from build123d import *

# Parameters (mm, degrees)
SKETCH1_R            = 3
SKETCH1_R_2          = 1.5
BOSS_EXTRUDE1_DEPTH  = 1.7
SKETCH4_W            = 49.75
SKETCH4_H            = 5.233449475
BOSS_EXTRUDE4_DEPTH  = 3
SKETCH7_W            = 6.5
SKETCH7_H            = 5.5
SKETCH7_W_2          = 7
SKETCH7_H_2          = 0.5
BOSS_EXTRUDE7_DEPTH  = 3
SKETCH8_W            = 13
SKETCH8_H            = 12
BOSS_EXTRUDE8_DEPTH  = 6.5
SKETCH9_W            = 5
SKETCH9_H            = 12
BOSS_EXTRUDE9_DEPTH  = 6
SKETCH10_W           = 20
SKETCH10_H           = 14
BOSS_EXTRUDE10_DEPTH = 13.5
SKETCH11_W           = 17
SKETCH11_H           = 12
BOSS_EXTRUDE11_DEPTH = 16
SKETCH12_W           = 10.053569384
SKETCH12_H           = 13.342225903
SKETCH12_W_2         = 14.279787724
SKETCH12_H_2         = 14.279787724
SKETCH12_W_3         = 9
SKETCH12_H_3         = 9
BOSS_EXTRUDE12_DEPTH = 2
SKETCH13_R           = 2.25
SKETCH13_R_2         = 1.5
BOSS_EXTRUDE13_DEPTH = 2
CUT_EXTRUDE1_DEPTH   = 9
CUT_EXTRUDE2_DEPTH   = 5
SKETCH16_W           = 11
SKETCH16_H           = 4
CUT_EXTRUDE3_DEPTH   = 10
SKETCH17_W           = 11
SKETCH17_H           = 4
CUT_EXTRUDE4_DEPTH   = 10
CUT_EXTRUDE5_DEPTH   = 12


with BuildPart() as part:
    # Sketch1 → Boss-Extrude1 (new body)
    with BuildSketch(Plane(origin=(0, 0, 0), x_dir=(1, 0, 0), z_dir=(0, 1, 0))):
        with BuildLine():
            ThreePointArc((39.5, 24.5), (41.621320344, 23.621320344), (42.5, 21.5))
            Line((42.5, 21.5), (42.5, -28.5))
            ThreePointArc((42.5, -28.5), (41.621320344, -30.621320344), (39.5, -31.5))
            Line((39.5, -31.5), (-39.5, -31.5))
            ThreePointArc((-39.5, -31.5), (-41.621320344, -30.621320344), (-42.5, -28.5))
            Line((-42.5, -28.5), (-42.5, 21.5))
            ThreePointArc((-42.5, 21.5), (-41.621320344, 23.621320344), (-39.5, 24.5))
            Line((-39.5, 24.5), (39.5, 24.5))
        make_face()
        with Locations((19, -28)):
            Circle(SKETCH1_R, mode=Mode.SUBTRACT)
        with Locations((19, 21)):
            Circle(SKETCH1_R, mode=Mode.SUBTRACT)
        with Locations((-39, -28)):
            Circle(SKETCH1_R, mode=Mode.SUBTRACT)
        with Locations((-39, 21)):
            Circle(SKETCH1_R, mode=Mode.SUBTRACT)
        with Locations((19, 21)):
            Circle(SKETCH1_R)
        with Locations((19, 21)):
            Circle(SKETCH1_R_2, mode=Mode.SUBTRACT)
        with Locations((-39, 21)):
            Circle(SKETCH1_R)
        with Locations((-39, 21)):
            Circle(SKETCH1_R_2, mode=Mode.SUBTRACT)
        with Locations((-39, -28)):
            Circle(SKETCH1_R)
        with Locations((-39, -28)):
            Circle(SKETCH1_R_2, mode=Mode.SUBTRACT)
        with Locations((19, -28)):
            Circle(SKETCH1_R)
        with Locations((19, -28)):
            Circle(SKETCH1_R_2, mode=Mode.SUBTRACT)
    extrude(amount=BOSS_EXTRUDE1_DEPTH)

    # Sketch4 → Boss-Extrude4 (add)
    with BuildSketch(Plane(origin=(0, 1.7, 0), x_dir=(1, 0, 0), z_dir=(0, 1, 0))):
        with Locations((-10, 21.068102783)):
            Rectangle(SKETCH4_W, SKETCH4_H)
    extrude(amount=BOSS_EXTRUDE4_DEPTH)

    # Sketch7 → Boss-Extrude7 (add)
    with BuildSketch(Plane(origin=(0, 1.7, 0), x_dir=(1, 0, 0), z_dir=(0, 1, 0))):
        with Locations((-31.9, -29.194183223)):
            Rectangle(SKETCH7_W, SKETCH7_H)
        with Locations((-31.9, -32.194183223)):
            Rectangle(SKETCH7_W_2, SKETCH7_H_2)
    extrude(amount=BOSS_EXTRUDE7_DEPTH)

    # Sketch8 → Boss-Extrude8 (add)
    with BuildSketch(Plane(origin=(0, 1.7, 0), x_dir=(1, 0, 0), z_dir=(0, 1, 0))):
        with Locations((-10.5, -26.626453528)):
            Rectangle(SKETCH8_W, SKETCH8_H)
    extrude(amount=BOSS_EXTRUDE8_DEPTH)

    # Sketch9 → Boss-Extrude9 (add)
    with BuildSketch(Plane(origin=(0, 1.7, 0), x_dir=(1, 0, 0), z_dir=(0, 1, 0))):
        with Locations((11, -25.5)):
            Rectangle(SKETCH9_W, SKETCH9_H)
    extrude(amount=BOSS_EXTRUDE9_DEPTH)

    # Sketch10 → Boss-Extrude10 (add)
    with BuildSketch(Plane(origin=(0, 1.7, 0), x_dir=(1, 0, 0), z_dir=(0, 1, 0))):
        with Locations((35, -21.25)):
            Rectangle(SKETCH10_W, SKETCH10_H)
    extrude(amount=BOSS_EXTRUDE10_DEPTH)

    # Sketch11 → Boss-Extrude11 (add)
    with BuildSketch(Plane(origin=(0, 1.7, 0), x_dir=(1, 0, 0), z_dir=(0, 1, 0))):
        with Locations((36.5, -2.5)):
            Rectangle(SKETCH11_W, SKETCH11_H)
        with Locations((36.5, 15.5)):
            Rectangle(SKETCH11_W, SKETCH11_H)
    extrude(amount=BOSS_EXTRUDE11_DEPTH)

    # Sketch12 → Boss-Extrude12 (add)
    with BuildSketch(Plane(origin=(0, 1.7, 0), x_dir=(1, 0, 0), z_dir=(0, 1, 0))):
        with Locations((-29.848215308, 10.97382243)):
            Rectangle(SKETCH12_W, SKETCH12_H)
        with Locations((-15.157331854, -3.918986484)):
            Rectangle(SKETCH12_W_2, SKETCH12_H_2)
        with Locations((19.1, -3.31)):
            Rectangle(SKETCH12_W_3, SKETCH12_H_3)
    extrude(amount=BOSS_EXTRUDE12_DEPTH)

    # Sketch13 → Boss-Extrude13 (add)
    with BuildSketch(Plane.XY.offset(31.5)):
        with Locations((11, 4.7)):
            Circle(SKETCH13_R)
        with Locations((11, 4.7)):
            Circle(SKETCH13_R_2, mode=Mode.SUBTRACT)
    extrude(amount=BOSS_EXTRUDE13_DEPTH)

    # Sketch14 → Cut-Extrude1 (cut)
    with BuildSketch(Plane.XY.offset(32.626453528)):
        with BuildLine():
            Line((-15.750323675, 5.983842352), (-4.86762122, 5.983842352))
            ThreePointArc((-4.86762122, 5.983842352), (-4.705559797, 5.901043441), (-4.677683467, 5.721203306))
            Line((-4.677683467, 5.721203306), (-5.276717124, 3.904778668))
            ThreePointArc((-5.276717124, 3.904778668), (-5.349453787, 3.805356292), (-5.466654877, 3.767417714))
            Line((-5.466654877, 3.767417714), (-15.151290018, 3.767417714))
            ThreePointArc((-15.151290018, 3.767417714), (-15.268491107, 3.805356292), (-15.341227771, 3.904778668))
            Line((-15.341227771, 3.904778668), (-15.940261428, 5.721203306))
            ThreePointArc((-15.940261428, 5.721203306), (-15.912385097, 5.901043441), (-15.750323675, 5.983842352))
        make_face()
    extrude(amount=-CUT_EXTRUDE1_DEPTH, mode=Mode.SUBTRACT)

    # Sketch15 → Cut-Extrude2 (cut)
    with BuildSketch(Plane.XY.offset(32.444183223)):
        with BuildLine():
            Line((-34.475250903, 3.20419671), (-29.43081526, 3.20419671))
            ThreePointArc((-29.43081526, 3.20419671), (-29.27664987, 3.131605628), (-29.234394805, 2.966527034))
            Line((-29.234394805, 2.966527034), (-29.471007813, 1.732759202))
            ThreePointArc((-29.471007813, 1.732759202), (-29.540019351, 1.616263488), (-29.667428269, 1.570428878))
            Line((-29.667428269, 1.570428878), (-34.24114908, 1.570428878))
            ThreePointArc((-34.24114908, 1.570428878), (-34.36870932, 1.616388672), (-34.437643137, 1.733145027))
            Line((-34.437643137, 1.733145027), (-34.67174496, 2.966912859))
            ThreePointArc((-34.67174496, 2.966912859), (-34.62929111, 3.13175695), (-34.475250903, 3.20419671))
        make_face()
    extrude(amount=-CUT_EXTRUDE2_DEPTH, mode=Mode.SUBTRACT)

    # Sketch16 → Cut-Extrude3 (cut)
    with BuildSketch(Plane(origin=(45, 0, 0), x_dir=(0, 0, -1), z_dir=(1, 0, 0))):
        with Locations((-2.5, 4.7)):
            Rectangle(SKETCH16_W, SKETCH16_H)
        with Locations((-2.5, 14.7)):
            Rectangle(SKETCH16_W, SKETCH16_H)
    extrude(amount=-CUT_EXTRUDE3_DEPTH, mode=Mode.SUBTRACT)

    # Sketch17 → Cut-Extrude4 (cut)
    with BuildSketch(Plane(origin=(45, 0, 0), x_dir=(0, 0, -1), z_dir=(1, 0, 0))):
        with Locations((15.5, 14.7)):
            Rectangle(SKETCH17_W, SKETCH17_H)
        with Locations((15.5, 4.7)):
            Rectangle(SKETCH17_W, SKETCH17_H)
    extrude(amount=-CUT_EXTRUDE4_DEPTH, mode=Mode.SUBTRACT)

    # Sketch18 → Cut-Extrude5 (cut)
    with BuildSketch(Plane(origin=(45, 0, 0), x_dir=(0, 0, -1), z_dir=(1, 0, 0))):
        Polygon((-26.75, 14), (-26.75, 3.95), (-23.25, 3.95), (-23.25, 1.95), (-19.25, 1.95), (-19.25, 3.95), (-15.75, 3.95), (-15.75, 14), align=None)
    extrude(amount=-CUT_EXTRUDE5_DEPTH, mode=Mode.SUBTRACT)


solid = part.part
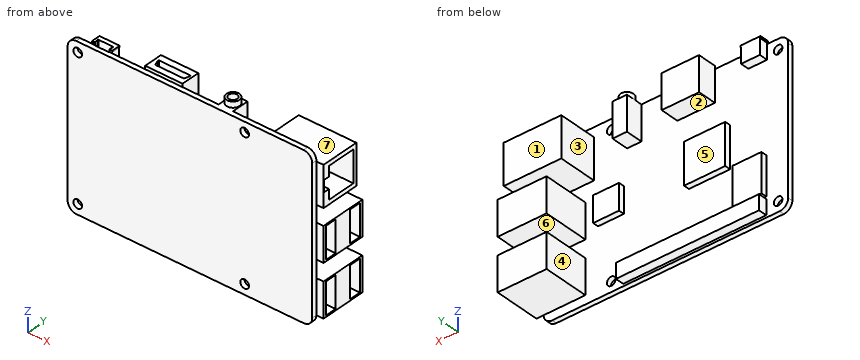
Geometry check sheet. Reference: the model listing, model coordinates, mm. Face numbers are marked on the shaded views. A direction names the side the tool comes from. Give positions to 0.01 mm unless a question says otherwise; leave off trailing zeros. Order: outer loops, then holes, each group sorted by start corner. A loop starts at its lowest first (then second) coordinate and runs counter-clockwise, first axis right, second up. Notation, with made-up numbers: (68, 35.25) - (84, 35.25) arc R16 ccw to (84, 42.25) - close; hole circle Ø3 at (37, 8.5). An arc over 180 degrees is marked (long way). Use one line per item in the form item = value.
1) Sectioned sample at A-A (y = 10.75). Record the boundary of the cut face in (x, z), and give its area (3 significant figures).
Working result:
outline = (25, 14.25) - (45, 14.25) - (45, 15.75) - (33, 15.75) - (33, 26.75) - (45, 26.75) - (45, 28.25) - (25, 28.25) - close; (28, -21.5) - (45, -21.5) - (45, -9.5) - (28, -9.5) - close; (28, -3.5) - (45, -3.5) - (45, 8.5) - (28, 8.5) - close
area = 556 mm^2
2) Sectioned sample at C-C (z = -8.5). Record the boundary of the cut face in (x, y) (3 decimals), and give its area (3 significant figures).
Working result:
outline = (-42.5, 0) - (42.5, 0) - (42.5, 1.7) - (-24.821, 1.7) - (-24.821, 3.7) - (-34.875, 3.7) - (-34.875, 1.7) - (-42.5, 1.7) - close
area = 165 mm^2
3) Depth check by flat-ended pin: pin 1 Ø4.5 at (x, z) = (-13, 2.5) entering from +Y; pin 2 Ø4.5 at (x, y) = (40, 14.5) entering from -Z; pin 3 Ø2 at (y, z) = (5.5, 1) entering from +X. Enter the tip coordinate at first touch or a pass-through.
Working result:
pin_1 = 3.7
pin_2 = -21.5
pin_3 = 35
4) Draft check along Z on the marked faces 4, 5, 6 and 7. Enter one of: released by +Z, released by -Z, zero draft, split by the parting line, or undercut.
Working result:
face_4 = zero draft
face_5 = undercut
face_6 = undercut
face_7 = released by +Z
5) Material ranges on probe 1 along Z at (x, y) = (-39, 0.65); probe 2 along Z at (x, y) = (40, 13); probe 3 along Z at (x, y) = (33, 15), recorded low to high. Write a range as from..to.
Working result:
probe_1 = -24.5..-22.5, -19.5..26.5, 29.5..31.5
probe_2 = -21.5..-21, -10..-9.5, -3.5..-3, 8..8.5, 14.25..15.75, 26.75..28.25
probe_3 = -21.5..-9.5, -3.5..8.5, 14.25..28.25
6) Sectioned sample at B-B (z = 24.5). Record the boundary of the cut face in (x, y).
Working result:
outline = (-42.5, 0) - (42.5, 0) - (42.5, 1.7) - (45, 1.7) - (45, 3.95) - (33, 3.95) - (33, 14) - (45, 14) - (45, 15.2) - (25, 15.2) - (25, 1.7) - (13.5, 1.7) - (13.5, 7.7) - (8.5, 7.7) - (8.5, 1.7) - (-4, 1.7) - (-4, 8.2) - (-17, 8.2) - (-17, 1.7) - (-42.5, 1.7) - close; hole (-15.94, 5.72) - (-15.34, 3.9) arc R0.2 ccw to (-15.15, 3.77) - (-5.47, 3.77) arc R0.2 ccw to (-5.28, 3.9) - (-4.68, 5.72) arc R0.2 ccw to (-4.87, 5.98) - (-15.75, 5.98) arc R0.2 ccw to start
7) Sectioned sample at D-D (x = 11). Record the boundary of the cut face in (y, z), and give its area (3 significant figures).
Working result:
outline = (0, -24.5) - (1.7, -24.5) - (1.7, -23.68) - (4.7, -23.68) - (4.7, -18.45) - (1.7, -18.45) - (1.7, 19.5) - (7.7, 19.5) - (7.7, 31.5) - (6.95, 31.5) - (6.95, 33.5) - (6.2, 33.5) - (6.2, 31.5) - (3.2, 31.5) - (3.2, 33.5) - (2.45, 33.5) - (2.45, 31.5) - (0, 31.5) - close
area = 186 mm^2
8) Access from +Z, -Z, +X, -X, +Y, -Y to the whole of each face (thin tool, end or side, straight path). Record for the marked faces 1, 2 and 3.
Working result:
face_1 = +Z, +X, -X, +Y
face_2 = -X, +Y
face_3 = +Z, -Z, +Y
